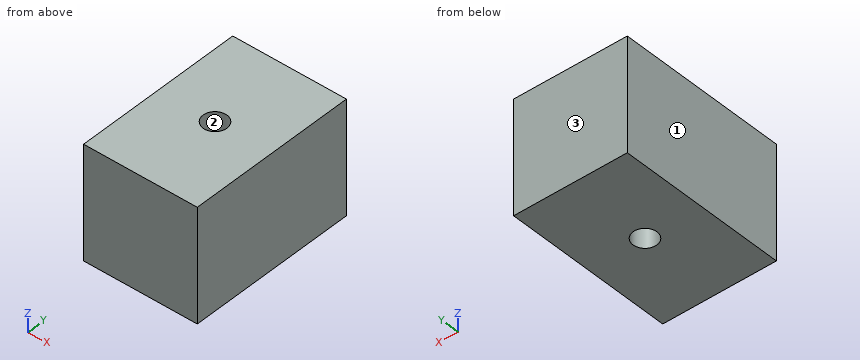
Autodesk Inventor part; units mm, degrees
ref_plane "YZ Plane" through (0, 0, 0) normal (1, 0, 0) x (0, 1, 0)
ref_plane "XZ Plane" through (0, 0, 0) normal (0, 1, 0) x (-1, 0, 0)
ref_plane "XY Plane" through (0, 0, 0) normal (0, 0, 1) x (1, 0, 0)
sketch "Sketch1" plane through (0, 0, 0) normal (0, 0, 1) x (1, 0, 0)
  line L0 (0, 0) -> (40, 0)
  line L1 (40, 0) -> (40, 60)
  line L2 (40, 60) -> (0, 60)
  line L3 (0, 60) -> (0, 0)
  dimension "d0" = 40
  dimension "d1" = 60
extrude "Extrusion1" add sketch "Sketch1" along normal blind 40
sketch "Sketch2" plane through (0, 0, 40) normal (0, 0, 1) x (1, 0, 0)
  circle A0 centre (20, 30) radius 6
  line L0 (0, 0) -> (40, 0)
  line L1 (40, 0) -> (40, 60)
  point P0 (20, 0)
  dimension "d4" = 12
  dimension "d12" = 30
  dimension "d13" = 20
hole "Hole1" at (20, 30, 40) direction (0, 0, -1) diameter 8.376 end through all
properties part number "Aluminium block"
Geometry check sheet. Reference: the model listing, model coordinates, mm. Face numbers are marked on the shaded views. Round coordinates to 2 decimals unless told otherwise and drop trailing zeros. Order: outer loops, then holes, each group sorted by start corner. A loop starts at its lowest first (then second) coordinate and runs counter-clockwise, first axis right, second up. Notation, with made-up numbers: (47, 8.25) - (85, 8.25) arc R22 ccw to (85, 29.25) - close; hole circle Ø7 at (75, 36.5). An arc over 180 degrees is marked (long way). Use a Markdown table: item, result. Add a question column.
1) Section check B-B (x = 20). Record the cut outline in (y, z), then the cut area to 3 significant figures.
2) Section check A-A (y = 30). Record the cut outline in (x, z), then the cut area to 3 significant figures.
3) Section check C-C (z = 30). Record the cut outline in (x, y), then the cut area to 3 significant figures.
4) Thickness scan on line 1 along X through (y, z) = (30, 16); line 2 along Y through (x, z) = (20, 29.5); line 3 along Y through (x, z) = (17, 31). Record the ranges inside material, lowest first.
5) Gauge pin test, flat end, axial feed: P1, Ø5, axis at x = 20, y = 30, coming from the -Z side. Record the tip position at first contact, or that the pin passes through.
6) Mould release check, pull along Y, two halves, no side actions. Record for the marked faces 1, 2 and 3: released by +Y, released by -Y, zero draft, split by the parting line, or undercut.
Established:
| question | item | result |
|---|---|---|
| 1 | outline | (0, 0) - (25.81, 0) - (25.81, 40) - (0, 40) - close; (34.19, 0) - (60, 0) - (60, 40) - (34.19, 40) - close |
| 1 | area | 2,060 mm2 |
| 2 | outline | (0, 0) - (15.81, 0) - (15.81, 40) - (0, 40) - close; (24.19, 0) - (40, 0) - (40, 40) - (24.19, 40) - close |
| 2 | area | 1,260 mm2 |
| 3 | outline | (0, 0) - (40, 0) - (40, 60) - (0, 60) - close; hole circle Ø8.38 at (20, 30) |
| 3 | area | 2,340 mm2 |
| 4 | line 1 | 0 to 15.81, 24.19 to 40 |
| 4 | line 2 | 0 to 25.81, 34.19 to 60 |
| 4 | line 3 | 0 to 27.08, 32.92 to 60 |
| 5 | P1 | through |
| 6 | face 1 | zero draft |
| 6 | face 2 | undercut |
| 6 | face 3 | released by +Y |
